Can you work these out from the drawing? Everything is in mm from the part's minimum corner. A direction names the side the tool comes from. Coordinates: 2 decimals unless noted, no trailing zeros. Loops run counter-clockwise (first coordinate to the right, second up) from the corner with the lowest first, then second, coordinate; pieces in that order, holes last. Notation, with made-up numbers: (68, 81) - (100, 81) arc R15 ccw to (100, 103) - close; hole circle Ø6 at (1.5, -27). An arc over 180 degrees is marked (long way). Put each result on its own line as item: value. Start each with the question number.
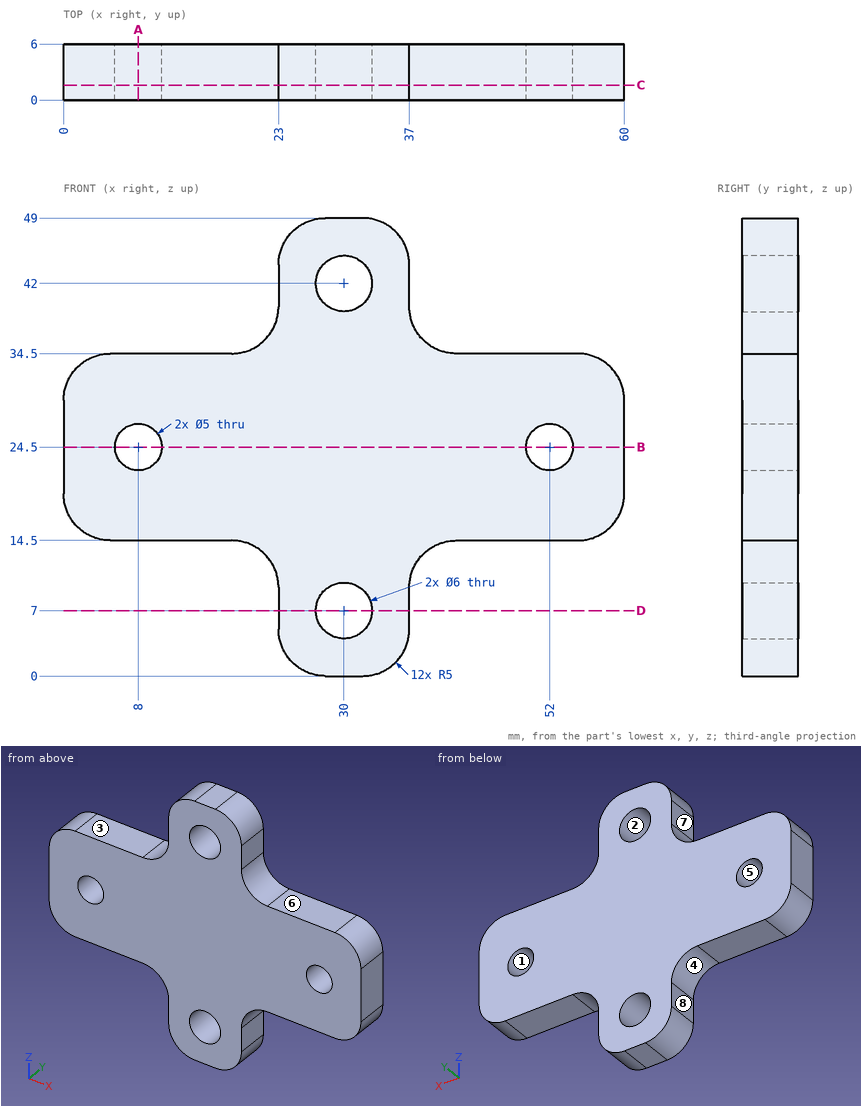
(1) For pin 1 Ø1.8 at (x, y) = (47, 2) entering from +Z; pin 2 Ø1.8 at (x, y) = (47.5, 2) entering from -Z; pin 3 Ø1.3 at (y, z) = (2, 42) entering from -X; pin 4 Ø4.5 at (x, z) = (52, 24.5) entering from -Y, each with a flat end and sliding along its axis, tell me the tip position at first contact or that it passes through.
(2) I need wall thicknesses on L1, parallel to Z at x = 30, y = 1.65; L2, parallel to Z at x = 52, y = 2.65; L3, parallel to Z at x = 27.5, y = 2.9. Which ranges of each line are inside material? Lowest first, please. Write a range as [from, to].
(3) If we mould it in two halves opening along X, with no side actions, what happens to the marked faces 1, 2, 3 and 4? For each: pulls with the +X half, pulls with the -X half, needs draft (parallel to the pull), parting line crosses it, or undercut.
(4) Which directions (+Z, -Z, +X, -X, +Y, -Y) give clear straight access to the entire face, cutting with the end or side of a thin tool? Please do the marked faces 5, 6, 7 and 8.
(5) I want a section at A-A on x = 8. List the corners of the cut face in (y, z) for me.
(6) I want a section at D-D on z = 7. List the corners of the cut face in (x, y) for me, and give its area (3 significant figures).
(7) I want a section at C-C on y = 1.6. List the corners of the cut face in (x, z) for me.
(8) I want a section at B-B on z = 24.5. List the corners of the cut face in (x, y) for me, and give its area (3 significant figures).
Answer sheet:
1. pin 1: stops at z = 34.5
1. pin 2: stops at z = 14.5
1. pin 3: stops at x = 23
1. pin 4: passes through
2. L1: z = [0, 4], [10, 39], [45, 49]
2. L2: z = [14.5, 22], [27, 34.5]
2. L3: z = [0.03, 5.34], [8.66, 40.34], [43.66, 48.97]
3. face 1: undercut
3. face 2: undercut
3. face 3: needs draft
3. face 4: pulls with the -X half
4. face 5: +Y, -Y
4. face 6: +Z, +X, +Y, -Y
4. face 7: +Z, -X, +Y, -Y
4. face 8: -Z, -X, +Y, -Y
5. outline: (0, 14.5) - (6, 14.5) - (6, 22) - (0, 22) - close; (0, 27) - (6, 27) - (6, 34.5) - (0, 34.5) - close
6. outline: (23, 0) - (27, 0) - (27, 6) - (23, 6) - close; (33, 0) - (37, 0) - (37, 6) - (33, 6) - close
6. area: 48.0 mm^2
7. outline: (0, 19.5) arc R5 ccw to (5, 14.5) - (18, 14.5) arc R5 cw to (23, 9.5) - (23, 5) arc R5 ccw to (28, 0) - (32, 0) arc R5 ccw to (37, 5) - (37, 9.5) arc R5 cw to (42, 14.5) - (55, 14.5) arc R5 ccw to (60, 19.5) - (60, 29.5) arc R5 ccw to (55, 34.5) - (42, 34.5) arc R5 cw to (37, 39.5) - (37, 44) arc R5 ccw to (32, 49) - (28, 49) arc R5 ccw to (23, 44) - (23, 39.5) arc R5 cw to (18, 34.5) - (5, 34.5) arc R5 ccw to (0, 29.5) - close; hole circle Ø5 at (8, 24.5); hole circle Ø6 at (30, 7); hole circle Ø6 at (30, 42); hole circle Ø5 at (52, 24.5)
8. outline: (0, 0) - (5.5, 0) - (5.5, 6) - (0, 6) - close; (10.5, 0) - (49.5, 0) - (49.5, 6) - (10.5, 6) - close; (54.5, 0) - (60, 0) - (60, 6) - (54.5, 6) - close
8. area: 300 mm^2
